Check sheet for the modelled part. Datum: model origin and axes. Units: mm. Face numbers are marked on the shaded views. A direction names the side the tool comes from. Coordinates: 2 decimals unless noted, no trailing zeros. Loops run counter-clockwise (first coordinate to the right, second up) from the corner with the lowest first, then second, coordinate; pieces in that order, holes last.
```python
from build123d import *

# Parameters (mm, degrees)
F3_R     = 3.05
F4_DEPTH = 6.75
F5_W     = 4.5
F5_H     = 2
F6_DEPTH = 5
F8_DEPTH = 12.5


with BuildPart() as f4:
    # F3 (on Front) → F4 (new body, symmetric)
    with BuildSketch(Plane.XZ):
        with BuildLine():
            ThreePointArc((3.8213217609, -1), (3.9176983648, -0.5041225271), (3.95, 0))
            ThreePointArc((3.95, 0), (3.9176983648, 0.5041225271), (3.8213217609, 1))
            Line((3.8213217609, 1), (3.05, 1))
            Line((3.05, 1), (3.05, 2.5))
            Line((3.05, 2.5), (3.0581857367, 2.5))
            ThreePointArc((3.0581857367, 2.5), (2.7930717857, 2.7930717857), (2.5, 3.0581857367))
            Line((2.5, 3.0581857367), (2.5, 3.05))
            Line((2.5, 3.05), (1, 3.05))
            Line((1, 3.05), (1, 3.8213217609))
            ThreePointArc((1, 3.8213217609), (0, 3.95), (-1, 3.8213217609))
            Line((-1, 3.8213217609), (-1, 3.05))
            Line((-1, 3.05), (-2.5, 3.05))
            Line((-2.5, 3.05), (-2.5, 3.0581857367))
            ThreePointArc((-2.5, 3.0581857367), (-2.7930717857, 2.7930717857), (-3.0581857367, 2.5))
            Line((-3.0581857367, 2.5), (-3.05, 2.5))
            Line((-3.05, 2.5), (-3.05, 1))
            Line((-3.05, 1), (-3.8213217609, 1))
            ThreePointArc((-3.8213217609, 1), (-3.95, 0), (-3.8213217609, -1))
            Line((-3.8213217609, -1), (-3.05, -1))
            Line((-3.05, -1), (-3.05, -2.5))
            Line((-3.05, -2.5), (-3.0581857367, -2.5))
            ThreePointArc((-3.0581857367, -2.5), (-2.7930717857, -2.7930717857), (-2.5, -3.0581857367))
            Line((-2.5, -3.0581857367), (-2.5, -3.05))
            Line((-2.5, -3.05), (-1, -3.05))
            Line((-1, -3.05), (-1, -3.8213217609))
            ThreePointArc((-1, -3.8213217609), (0, -3.95), (1, -3.8213217609))
            Line((1, -3.8213217609), (1, -3.05))
            Line((1, -3.05), (2.5, -3.05))
            Line((2.5, -3.05), (2.5, -3.0581857367))
            ThreePointArc((2.5, -3.0581857367), (2.7930717857, -2.7930717857), (3.0581857367, -2.5))
            Line((3.0581857367, -2.5), (3.05, -2.5))
            Line((3.05, -2.5), (3.05, -1))
            Line((3.05, -1), (3.8213217609, -1))
        make_face()
        Circle(F3_R, mode=Mode.SUBTRACT)
        with BuildLine():
            Line((3.05, 1), (3.8213217609, 1))
            ThreePointArc((3.8213217609, 1), (3.5205689671, 1.7911153363), (3.0581857367, 2.5))
            Line((3.0581857367, 2.5), (3.05, 2.5))
            Line((3.05, 2.5), (3.05, 1))
        make_face()
        with BuildLine():
            ThreePointArc((3.0581857367, 2.5), (3.5205689671, 1.7911153363), (3.8213217609, 1))
            Line((3.8213217609, 1), (5.95, 1))
            Line((5.95, 1), (5.95, 2.5))
            Line((5.95, 2.5), (3.0581857367, 2.5))
        make_face()
        with BuildLine():
            Line((5.95, -1), (3.8213217609, -1))
            ThreePointArc((3.8213217609, -1), (3.5205689671, -1.7911153363), (3.0581857367, -2.5))
            Line((3.0581857367, -2.5), (5.95, -2.5))
            Line((5.95, -2.5), (5.95, -1))
        make_face()
        with BuildLine():
            ThreePointArc((3.0581857367, -2.5), (3.5205689671, -1.7911153363), (3.8213217609, -1))
            Line((3.8213217609, -1), (3.05, -1))
            Line((3.05, -1), (3.05, -2.5))
            Line((3.05, -2.5), (3.0581857367, -2.5))
        make_face()
        with BuildLine():
            Line((2.5, 3.05), (2.5, 3.0581857367))
            ThreePointArc((2.5, 3.0581857367), (1.7911153363, 3.5205689671), (1, 3.8213217609))
            Line((1, 3.8213217609), (1, 3.05))
            Line((1, 3.05), (2.5, 3.05))
        make_face()
        with BuildLine():
            ThreePointArc((1, 3.8213217609), (1.7911153363, 3.5205689671), (2.5, 3.0581857367))
            Line((2.5, 3.0581857367), (2.5, 5.95))
            Line((2.5, 5.95), (1, 5.95))
            Line((1, 5.95), (1, 3.8213217609))
        make_face()
        with BuildLine():
            Line((2.5, -5.95), (2.5, -3.0581857367))
            ThreePointArc((2.5, -3.0581857367), (1.7911153363, -3.5205689671), (1, -3.8213217609))
            Line((1, -3.8213217609), (1, -5.95))
            Line((1, -5.95), (2.5, -5.95))
        make_face()
        with BuildLine():
            ThreePointArc((1, -3.8213217609), (1.7911153363, -3.5205689671), (2.5, -3.0581857367))
            Line((2.5, -3.0581857367), (2.5, -3.05))
            Line((2.5, -3.05), (1, -3.05))
            Line((1, -3.05), (1, -3.8213217609))
        make_face()
        with BuildLine():
            Line((-1, 3.05), (-1, 3.8213217609))
            ThreePointArc((-1, 3.8213217609), (-1.7911153363, 3.5205689671), (-2.5, 3.0581857367))
            Line((-2.5, 3.0581857367), (-2.5, 3.05))
            Line((-2.5, 3.05), (-1, 3.05))
        make_face()
        with BuildLine():
            ThreePointArc((-2.5, 3.0581857367), (-1.7911153363, 3.5205689671), (-1, 3.8213217609))
            Line((-1, 3.8213217609), (-1, 5.95))
            Line((-1, 5.95), (-2.5, 5.95))
            Line((-2.5, 5.95), (-2.5, 3.0581857367))
        make_face()
        with BuildLine():
            Line((-1, -5.95), (-1, -3.8213217609))
            ThreePointArc((-1, -3.8213217609), (-1.7911153363, -3.5205689671), (-2.5, -3.0581857367))
            Line((-2.5, -3.0581857367), (-2.5, -5.95))
            Line((-2.5, -5.95), (-1, -5.95))
        make_face()
        with BuildLine():
            ThreePointArc((-2.5, -3.0581857367), (-1.7911153363, -3.5205689671), (-1, -3.8213217609))
            Line((-1, -3.8213217609), (-1, -3.05))
            Line((-1, -3.05), (-2.5, -3.05))
            Line((-2.5, -3.05), (-2.5, -3.0581857367))
        make_face()
        with BuildLine():
            Line((-3.05, 2.5), (-3.0581857367, 2.5))
            ThreePointArc((-3.0581857367, 2.5), (-3.5205689671, 1.7911153363), (-3.8213217609, 1))
            Line((-3.8213217609, 1), (-3.05, 1))
            Line((-3.05, 1), (-3.05, 2.5))
        make_face()
        with BuildLine():
            ThreePointArc((-3.8213217609, 1), (-3.5205689671, 1.7911153363), (-3.0581857367, 2.5))
            Line((-3.0581857367, 2.5), (-5.95, 2.5))
            Line((-5.95, 2.5), (-5.95, 1))
            Line((-5.95, 1), (-3.8213217609, 1))
        make_face()
        with BuildLine():
            Line((-5.95, -2.5), (-3.0581857367, -2.5))
            ThreePointArc((-3.0581857367, -2.5), (-3.5205689671, -1.7911153363), (-3.8213217609, -1))
            Line((-3.8213217609, -1), (-5.95, -1))
            Line((-5.95, -1), (-5.95, -2.5))
        make_face()
        with BuildLine():
            ThreePointArc((-3.8213217609, -1), (-3.5205689671, -1.7911153363), (-3.0581857367, -2.5))
            Line((-3.0581857367, -2.5), (-3.05, -2.5))
            Line((-3.05, -2.5), (-3.05, -1))
            Line((-3.05, -1), (-3.8213217609, -1))
        make_face()
    extrude(amount=F4_DEPTH, both=True)

    # F5 (on Right) → F6 (cut, symmetric)
    with BuildSketch(Plane.YZ):
        with Locations((-4.5, 0)):
            Rectangle(F5_W, F5_H)
        with Locations((4.5, 0)):
            Rectangle(F5_W, F5_H)
        with BuildLine():
            ThreePointArc((2.25, 1), (1.25, 0), (2.25, -1))
            Line((2.25, -1), (2.25, 1))
        make_face()
    extrude(amount=F6_DEPTH, both=True, mode=Mode.SUBTRACT)

    # F7 (on Top) → F8 (cut, symmetric)
    with BuildSketch(Plane.XY):
        with BuildLine():
            ThreePointArc((-1, -2.25), (0, -3.25), (1, -2.25))
            Line((1, -2.25), (1, 2.25))
            Line((1, 2.25), (-1, 2.25))
            Line((-1, 2.25), (-1, -2.25))
        make_face()
    extrude(amount=F8_DEPTH, both=True, mode=Mode.SUBTRACT)


solid = f4.part
```
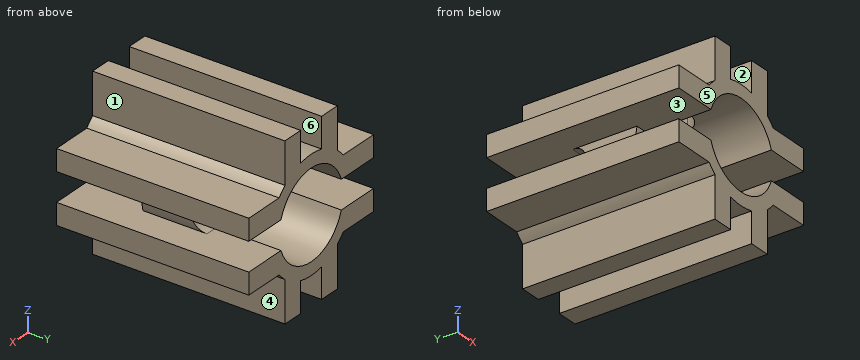
1) Depth check by flat-ended pin: pin 1 (3.5 mm diameter, centred on y = -1.5, z = 5, fed in from +X); pin 2 (2.5 mm diameter, centred on x = 5, y = -0.5, fed in from +Z); pin 3 (0.9 mm diameter, centred on x = 4, y = 0.5, fed in from -Z). Enter the tip coordinate at first touch or a pass-through.
Answer sheet:
pin 1: stops at x = 2.5
pin 2: stops at z = 2.5
pin 3: stops at z = -2.5
2) Scan lines: line 1 (X direction, y = 3.5, z = -1.75); line 2 (X direction, y = -0.25, z = 0); line 3 (Z direction, x = -3.75, y = -4.25). Record each from-to range of solid material in increasing order.
Answer sheet:
line 1: x = -5.95 to -2.5, 2.5 to 5.95
line 2: x = -3.95 to -3.05, 3.05 to 3.95
line 3: z = -2.5 to -1, 1 to 2.5
3) Set-up check for the marked faces 1, 2 and 3: record each of +Z, -Z, +X, -X, +Y, -Y from which the full face is reachable in a straight line by a thin tool's end or side.
Answer sheet:
face 1: +Z, +X, +Y, -Y
face 2: +Z
face 3: -X
4) Section check A-A on x = 4.5. Enter the section's corners in (y, z).
Answer sheet:
outline: (-6.75, -2.5) - (6.75, -2.5) - (6.75, -1) - (-6.75, -1) - close; (-6.75, 1) - (6.75, 1) - (6.75, 2.5) - (-6.75, 2.5) - close
5) Section check D-D on x = 0. Enter the section's corners in (y, z).
Answer sheet:
outline: (-6.75, -3.95) - (-3.25, -3.95) - (-3.25, -3.05) - (-6.75, -3.05) - close; (-6.75, 3.05) - (-3.25, 3.05) - (-3.25, 3.95) - (-6.75, 3.95) - close; (2.25, -3.95) - (6.75, -3.95) - (6.75, -3.05) - (2.25, -3.05) - close; (2.25, 3.05) - (6.75, 3.05) - (6.75, 3.95) - (2.25, 3.95) - close
6) Section check B-B on z = 0. Enter the section's corners in (x, y), plus the area to 3 significant figures.
Answer sheet:
outline: (-3.95, -2.25) - (-3.05, -2.25) - (-3.05, 1.25) - (-3.95, 1.25) - close; (3.05, -2.25) - (3.95, -2.25) - (3.95, 1.25) - (3.05, 1.25) - close
area: 6.30 mm2
7) Mould release check, pull along Y, two halves, no side actions. Record for the marked faces 4, 5 and 6: +Y half, -Y half, draft (parallel to the pull), parting line (faces both ways), or undercut.
Answer sheet:
face 4: draft
face 5: -Y half
face 6: undercut
